Answer from the drawing. Dimensions are ordinates in mm from the lowest x, y and z of the part. A direction names the side the tool comes from. Coordinates: 2 decimals unless noted, no trailing zeros. Order: outer loops, then holes, each group sorted by start corner. A loop starts at its lowest first (then second) coordinate and runs counter-clockwise, first axis right, second up. Notation, with made-up numbers: M 76.25,75 L 132.25,75 A15 cw 132.25,92 Z; hole C 57.25,-9.75 d6. An arc over 180 degrees is marked long. Use a Markdown table: item, result.
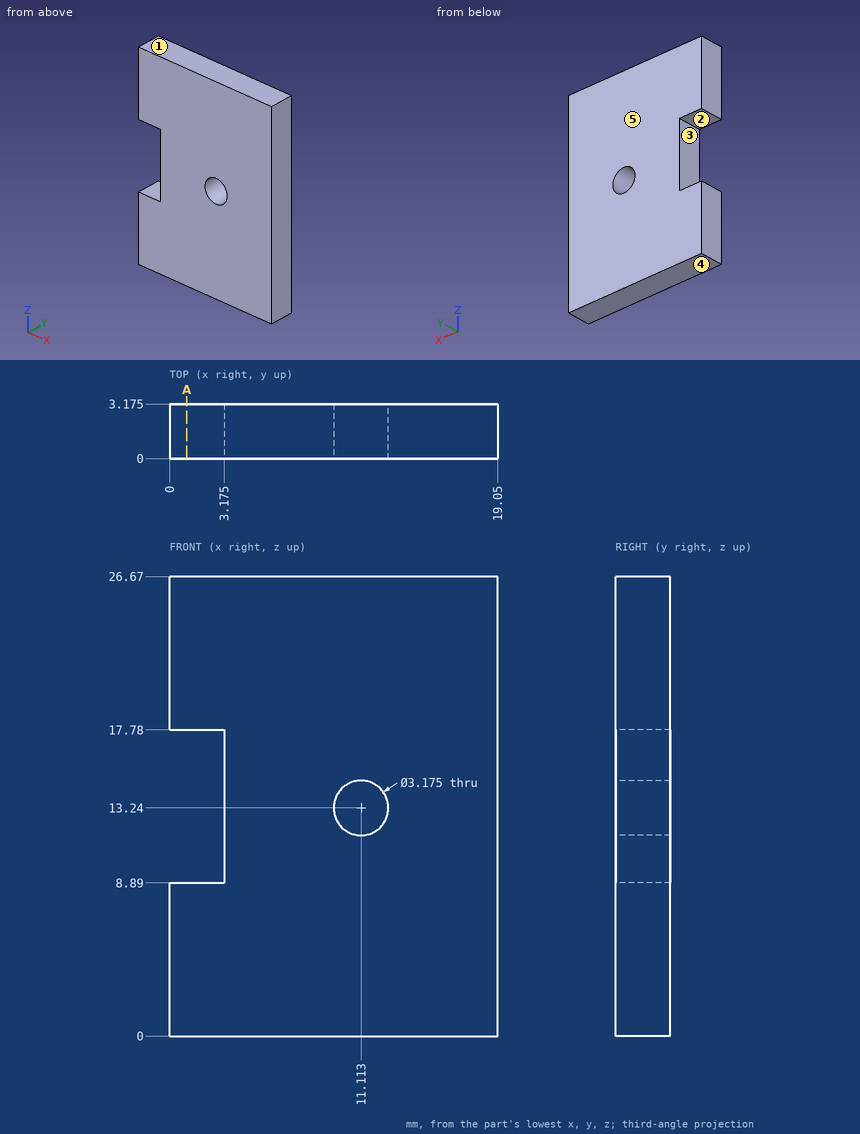
(1) A cutting plane is placed at A-A (x = 1). Determine the outline of the cut face in (y, z) (1 decimal).
Conclusion:
| item | result |
|---|---|
| outline | M 0,0 L 3.2,0 L 3.2,8.9 L 0,8.9 Z; M 0,17.8 L 3.2,17.8 L 3.2,26.7 L 0,26.7 Z |
(2) Determine the mould class of the marked faces 3, 4 and 5 for opening direction Z: pulls with the +Z half, pulls with the -Z half, needs draft (parallel to the pull), parting line crosses it, or undercut.
Conclusion:
| item | result |
|---|---|
| face 3 | undercut |
| face 4 | pulls with the -Z half |
| face 5 | needs draft |
(3) A straight line is drawn through the part: L1, parallel to Z at x = 11, y = 1.95. Find the intervals that lie inside material, in ascending order.
Conclusion:
| item | result |
|---|---|
| L1 | 0 to 11.66, 14.82 to 26.67 |
(4) Which of the six approach directions +Z, -Z, +X, -X, +Y, -Y give full straight-line access (tool end or side, diameter ignored) to the marked faces 1 and 2?
Conclusion:
| item | result |
|---|---|
| face 1 | +Z, +X, -X, +Y, -Y |
| face 2 | -X, +Y, -Y |
